Build history of the part. All positions in model axes, mm. Face numbers are marked on the shaded views. A direction names the side the tool comes from. Give positions to 0.01 mm unless a question says otherwise; leave off trailing zeros. Order: outer loops, then holes, each group sorted by start corner. A loop starts at its lowest first (then second) coordinate and runs counter-clockwise, first axis right, second up. Notation, with made-up numbers: (68, -15.75) -> (94, -15.75) arc R37 cw to (94, 20.25) -> close; hole circle Ø10 at (68, 76.5). An arc over 180 degrees is marked (long way). Write item = value, one per line. Start each with the question number.
from build123d import *

# Parameters (mm, degrees)
F0_W     = 342.9
F0_H     = 342.9
F1_DEPTH = 38.1
F0_W_2   = 38.1
F0_H_2   = 146.685
F0_H_3   = 38.1
F0_W_3   = 146.685
F2_DEPTH = 25.4


with BuildPart() as f1:
    # F0 (on Front) → F1 (new body)
    with BuildSketch(Plane.XZ):
        Rectangle(F0_W, F0_H)
        Polygon((127.635, 165.735), (165.735, 165.735), (165.735, 127.635), (165.735, 19.05), (165.735, -19.05), (165.735, -127.635), (165.735, -165.735), (127.635, -165.735), (19.05, -165.735), (-19.05, -165.735), (-127.635, -165.735), (-165.735, -165.735), (-165.735, -127.635), (-165.735, -19.05), (-165.735, 19.05), (-165.735, 127.635), (-165.735, 165.735), (-127.635, 165.735), (-19.05, 165.735), (19.05, 165.735), align=None, mode=Mode.SUBTRACT)
    extrude(amount=F1_DEPTH)

    # F0 (on Front) → F2 (join)
    with BuildSketch(Plane.XZ):
        with Locations((0, 92.3925)):
            Rectangle(F0_W_2, F0_H_2)
        with Locations((146.685, -146.685)):
            Rectangle(F0_W_2, F0_H_3)
        Rectangle(F0_W_2, F0_H_3)
        with Locations((146.685, 146.685)):
            Rectangle(F0_W_2, F0_H_3)
        with Locations((-92.3925, 0)):
            Rectangle(F0_W_3, F0_H_3)
        with Locations((92.3925, 0)):
            Rectangle(F0_W_3, F0_H_3)
        with Locations((-146.685, -146.685)):
            Rectangle(F0_W_2, F0_H_3)
        with Locations((0, -92.3925)):
            Rectangle(F0_W_2, F0_H_2)
        with Locations((-146.685, 146.685)):
            Rectangle(F0_W_2, F0_H_3)
    extrude(amount=F2_DEPTH)


solid = f1.part
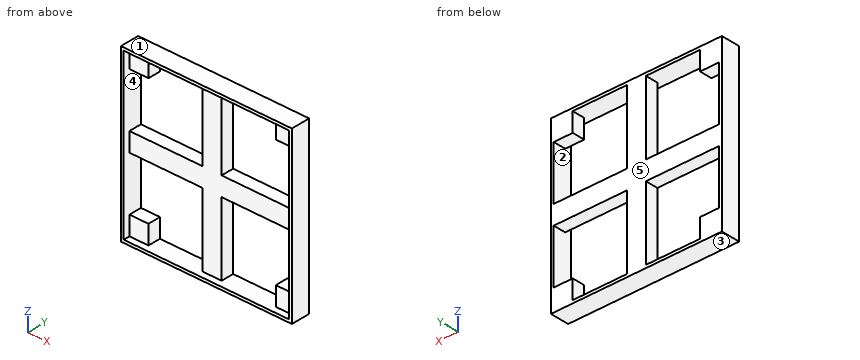
(1) Wall check: line 1 (Z direction, x = 121.5, y = -5) (3 decimals); line 2 (X direction, y = -15, z = -138) (3 decimals). Give the ranges that are in metal, low to high. Write a range as [from, to].
(2) Cut at C-C, the plane y = -11.5. Give the cut face in (x, z) (3 decimals), plus the area to 3 significant figures.
(3) Cut at A-A, the plane z = 120. Give the cut face in (x, y) (3 decimals).
(4) 3-axis set-ups, long thin cutter, end or side, ignore diameter. For the marked faces 4 and 5: which of +Z, -Z, +X, -X, +Y, -Y reach the whole face in a straight line?
(5) Cut at D-D, the plane z = 5. Give the cut face in (x, y) (3 decimals).
(6) Flat gauge pin, fed straight in: P1, Ø11.5, axis at x = 150.5, z = 152.5, coming from the -Y side. Where does the tip first touch, or does it go through?
(7) Cut at B-B, the plane x = -64. Give the cut face in (y, z) (3 decimals).
(8) Mould opens along Z. For the marked faces 1, 2 and 3 say: released by +Z, released by -Z, zero draft, split by the parting line, or undercut.
Results:
q1.line_1 = [-171.45, -165.735], [-19.05, 19.05], [165.735, 171.45]
q1.line_2 = [-171.45, -127.635], [-19.05, 19.05], [127.635, 171.45]
q2.outline = (-171.45, -171.45) -> (171.45, -171.45) -> (171.45, 171.45) -> (-171.45, 171.45) -> close; hole (-165.735, -127.635) -> (-127.635, -127.635) -> (-127.635, -165.735) -> (-19.05, -165.735) -> (-19.05, -19.05) -> (-165.735, -19.05) -> close; hole (-165.735, 19.05) -> (-19.05, 19.05) -> (-19.05, 165.735) -> (-127.635, 165.735) -> (-127.635, 127.635) -> (-165.735, 127.635) -> close; hole (19.05, -165.735) -> (127.635, -165.735) -> (127.635, -127.635) -> (165.735, -127.635) -> (165.735, -19.05) -> (19.05, -19.05) -> close; hole (19.05, 19.05) -> (165.735, 19.05) -> (165.735, 127.635) -> (127.635, 127.635) -> (127.635, 165.735) -> (19.05, 165.735) -> close
q2.area = 37,300 mm2
q3.outline = (-171.45, -38.1) -> (-165.735, -38.1) -> (-165.735, 0) -> (-171.45, 0) -> close; (-19.05, -25.4) -> (19.05, -25.4) -> (19.05, 0) -> (-19.05, 0) -> close; (165.735, -38.1) -> (171.45, -38.1) -> (171.45, 0) -> (165.735, 0) -> close
q4.face_4 = -Y
q4.face_5 = +Z, -Z, +X, -X, +Y
q5.outline = (-171.45, -38.1) -> (-165.735, -38.1) -> (-165.735, -25.4) -> (165.735, -25.4) -> (165.735, -38.1) -> (171.45, -38.1) -> (171.45, 0) -> (-171.45, 0) -> close
q6.P1 = -25.4
q7.outline = (-38.1, -171.45) -> (0, -171.45) -> (0, -165.735) -> (-38.1, -165.735) -> close; (-38.1, 165.735) -> (0, 165.735) -> (0, 171.45) -> (-38.1, 171.45) -> close; (-25.4, -19.05) -> (0, -19.05) -> (0, 19.05) -> (-25.4, 19.05) -> close
q8.face_1 = released by +Z
q8.face_2 = undercut
q8.face_3 = released by -Z
